Build history of the part. All positions in model axes, mm. Give positions to 0.01 mm unless a question says otherwise; leave off trailing zeros. Order: outer loops, then holes, each group sorted by start corner. A loop starts at its lowest first (then second) coordinate and runs counter-clockwise, first axis right, second up. Notation, with made-up numbers: (-26, -2.5) - (12, -2.5) arc R4 cw to (12, 1.5) - close; hole circle Ø8 at (-9, -1). An arc over 180 degrees is marked (long way). Use a Markdown table: item, result.
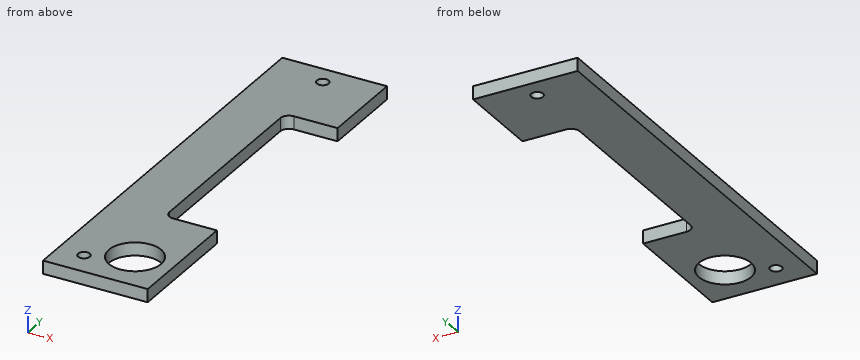
from build123d import *

# Parameters (mm, degrees)
BOSS_EXTRUDE1_DEPTH         = 4.7625
F_6_CLEARANCE_HOLE1_D       = 4.3053
F_3_4_0_75_DIAMETER_HOLE1_D = 19.05


with BuildPart() as part:
    # Sketch1 → Boss-Extrude1 (new body)
    with BuildSketch(Plane.XY):
        with BuildLine():
            Line((0, 44.45), (-15.875, 44.45))
            ThreePointArc((-15.875, 44.45), (-18.12006403, 45.37993597), (-19.05, 47.625))
            Line((-19.05, 47.625), (-19.05, 118.745))
            ThreePointArc((-19.05, 118.745), (-18.12006403, 120.99006403), (-15.875, 121.92))
            Line((-15.875, 121.92), (0, 121.92))
            Line((0, 121.92), (0, 153.67))
            Line((0, 153.67), (-38.1, 153.67))
            Line((-38.1, 153.67), (-38.1, 0))
            Line((-38.1, 0), (0, 0))
            Line((0, 0), (0, 44.45))
        make_face()
    extrude(amount=-BOSS_EXTRUDE1_DEPTH)

    # #6 Clearance Hole1 (through all)
    with Locations(Plane(origin=(0, 0, -4.7625), x_dir=(-1, 0, 0), z_dir=(0, 0, -1))):
        with Locations((28.575, 9.525), (19.05, 146.05)):
            Hole(F_6_CLEARANCE_HOLE1_D / 2)

    # 3/4 (0.75) Diameter Hole1 (through all)
    with Locations(Plane(origin=(0, 0, -4.7625), x_dir=(-1, 0, 0), z_dir=(0, 0, -1))):
        with Locations((13.97, 16.51)):
            Hole(F_3_4_0_75_DIAMETER_HOLE1_D / 2)


solid = part.part
1) Slice it at A-A (y = 16.51). Write the cut outline in (x, z) (1 decimal).
Computed:
| item | result |
|---|---|
| outline | (-38.1, -4.8) - (-23.5, -4.8) - (-23.5, 0) - (-38.1, 0) - close; (-4.4, -4.8) - (0, -4.8) - (0, 0) - (-4.4, 0) - close |
2) Slice it at B-B (x = -13.97). State how many separate pieces and enclosed holes the cut face has, and give its area (3 significant figures).
Computed:
| item | result |
|---|---|
| separate pieces | 3 |
| enclosed holes | 0 |
| area | 272 mm² |
3) Slice it at D-D (z = -3.75). Write the cut outline in (x, y) (3 decimals), and give its area (3 significant figures).
Computed:
| item | result |
|---|---|
| outline | (-38.1, 0) - (0, 0) - (0, 44.45) - (-15.875, 44.45) arc R3.175 cw to (-19.05, 47.625) - (-19.05, 118.745) arc R3.175 cw to (-15.875, 121.92) - (0, 121.92) - (0, 153.67) - (-38.1, 153.67) - close; hole circle Ø4.305 at (-28.575, 9.525); hole circle Ø19.05 at (-13.97, 16.51); hole circle Ø4.305 at (-19.05, 146.05) |
| area | 4,070 mm² |
4) Pin check, flat tip, straight feed: P1, Ø1.4, axis at y = 88.5, z = -3, coming from the +X side. Stop position of the tip, or through.
Computed:
| item | result |
|---|---|
| P1 | stops at x = -19.05 |
5) Slice it at C-C (y = 146.05). Write the cut outline in (x, z).
Computed:
| item | result |
|---|---|
| outline | (-38.1, -4.76) - (-21.2, -4.76) - (-21.2, 0) - (-38.1, 0) - close; (-16.9, -4.76) - (0, -4.76) - (0, 0) - (-16.9, 0) - close |
6) Wall check: line 1 (Y direction, x = -13.97, z = -1) (3 decimals); line 2 (X direction, y = 146.05, z = -2.35); line 3 (X direction, y = 17, z = -0.45). Give the ranges that are in metal, low to high. Write a range as from..to.
Computed:
| item | result |
|---|---|
| line 1 | y = 0..6.985, 26.035..44.45, 121.92..153.67 |
| line 2 | x = -38.1..-21.2, -16.9..0 |
| line 3 | x = -38.1..-23.48, -4.46..0 |
